Source: CAD feature listing. Evaluate the final solid. Frame: model axes, mm. A direction names the side the tool comes from. Coordinates: 2 decimals unless noted, no trailing zeros. Order: outer loops, then holes, each group sorted by start corner. A loop starts at its lowest first (then second) coordinate and runs counter-clockwise, first axis right, second up. Notation, with made-up numbers: (82, -23) - (130, -23) arc R34 cw to (130, 11) - close; hole circle Ø4 at (0.25, 81.5). An arc over 180 degrees is marked (long way). One line per question, with ' | ' between items.
from build123d import *

# Parameters (mm, degrees)
BASE_FLANGE1_DEPTH           = 150
F_30_0_1285_DIAMETER_HOLE1_D = 3.2639
FILLET1_R                    = 5


# Sheet-metal steps are written as plain solids
with BuildPart() as part:
    # Sketch1 → Base-Flange1 (new body)
    with BuildSketch(Plane.XY):
        with BuildLine():
            Line((-25.4, 0), (-6, 0))
            ThreePointArc((-6, 0), (-1.757359313, 1.757359313), (0, 6))
            Line((0, 6), (0, 50.8))
            Line((0, 50.8), (-3, 50.8))
            Line((-3, 50.8), (-3, 6))
            ThreePointArc((-3, 6), (-3.878679656, 3.878679656), (-6, 3))
            Line((-6, 3), (-25.4, 3))
            Line((-25.4, 3), (-25.4, 0))
        make_face()
    extrude(amount=BASE_FLANGE1_DEPTH)

    # #30 (0.1285) Diameter Hole1 (through all)
    with Locations(Plane(origin=(0, 3, 0), x_dir=(1, 0, 0), z_dir=(0, 1, 0))):
        with Locations((-15.7, -25), (-15.7, -75), (-15.7, -125)):
            Hole(F_30_0_1285_DIAMETER_HOLE1_D / 2)

    # Fillet1
    fillet1_edges = [part.edges().sort_by_distance(p)[0] for p in [
        (-1.5, 50.8, 150),
        (-1.5, 50.8, 0),
        (-25.4, 1.5, 150),
        (-25.4, 1.5, 0),
    ]]
    fillet(fillet1_edges, radius=FILLET1_R)


solid = part.part
(1) Pull-direction query (X, two-part tool) for faces 1 (the cylindrical face through (-15.346, 1.479, 26.593)), 2 (the flat face through (0, 28, 74)), 3 (the flat face through (-2.7, 16.2, 0)); classes: pulls with the +X half, pulls with the -X half, needs draft (parallel to the pull), parting line crosses it, or undercut.
Taken from the geometry:
face 1: undercut | face 2: pulls with the +X half | face 3: needs draft
(2) Set-up query: faces 4 (the flat face through (-3, 29, 74)), 5 (the cylindrical face through (-15.49, 1.48, 123.38)). Return all of +Z, -Z, +X, -X, +Y, -Y with unobstructed straight access to the full face (end or side cutting, diameter ignored); none if empty.
Taken from the geometry:
face 4: +Z, -Z, -X, +Y | face 5: +Y, -Y
(3) Cut plane C-C (z = 41). Return the cut outline in (x, y).
Taken from the geometry:
outline: (-25.4, 0) - (-6, 0) arc R6 ccw to (0, 6) - (0, 50.8) - (-3, 50.8) - (-3, 6) arc R3 cw to (-6, 3) - (-25.4, 3) - close
(4) Cut plane A-A (z = 25). Return the cut outline in (x, y).
Taken from the geometry:
outline: (-25.4, 0) - (-17.33, 0) - (-17.33, 3) - (-25.4, 3) - close; (-14.07, 0) - (-6, 0) arc R6 ccw to (0, 6) - (0, 50.8) - (-3, 50.8) - (-3, 6) arc R3 cw to (-6, 3) - (-14.07, 3) - close
(5) Cut plane B-B (x = -15.7). Return the cut outline in (y, z), and give its area (3 significant figures).
Taken from the geometry:
outline: (0, 0) - (3, 0) - (3, 23.37) - (0, 23.37) - close; (0, 26.63) - (3, 26.63) - (3, 73.37) - (0, 73.37) - close; (0, 76.63) - (3, 76.63) - (3, 123.37) - (0, 123.37) - close; (0, 126.63) - (3, 126.63) - (3, 150) - (0, 150) - close | area: 421 mm²
(6) Cut plane D-D (y = 36). Return the cut outline in (x, z), and give its area (3 significant figures).
Taken from the geometry:
outline: (-3, 0) - (0, 0) - (0, 150) - (-3, 150) - close | area: 450 mm²
(7) Pin query (flat end, axial travel): P1, Ø1.5, axis at y = 42.5, z = 42.5, coming from the -X side; P2, Ø6, axis at x = -13.5, z = 77.5, coming from the +Y side. Return the tip coordinate at first contact, or that it passes through.
Taken from the geometry:
P1: stops at x = -3 | P2: stops at y = 3
(8) Material intervals for L1, parallel to Z at x = -15.7, y = 1.1; L2, parallel to X at y = 19, z = 14.5; L3, parallel to Y at x = -20, z = 38, sorted ascending. Write a range as from..to.
Taken from the geometry:
L1: z = 0..23.37, 26.63..73.37, 76.63..123.37, 126.63..150 | L2: x = -3..0 | L3: y = 0..3
